Answer from the drawing. Dimensions are ordinates in mm from the lowest x, y and z of the part. Give positions to 0.01 mm unless a question says otherwise; leave off trailing zeros. Order: outer loops, then holes, each group sorted by start corner. A loop starts at its lowest first (then second) coordinate and runs counter-clockwise, first axis right, second up.
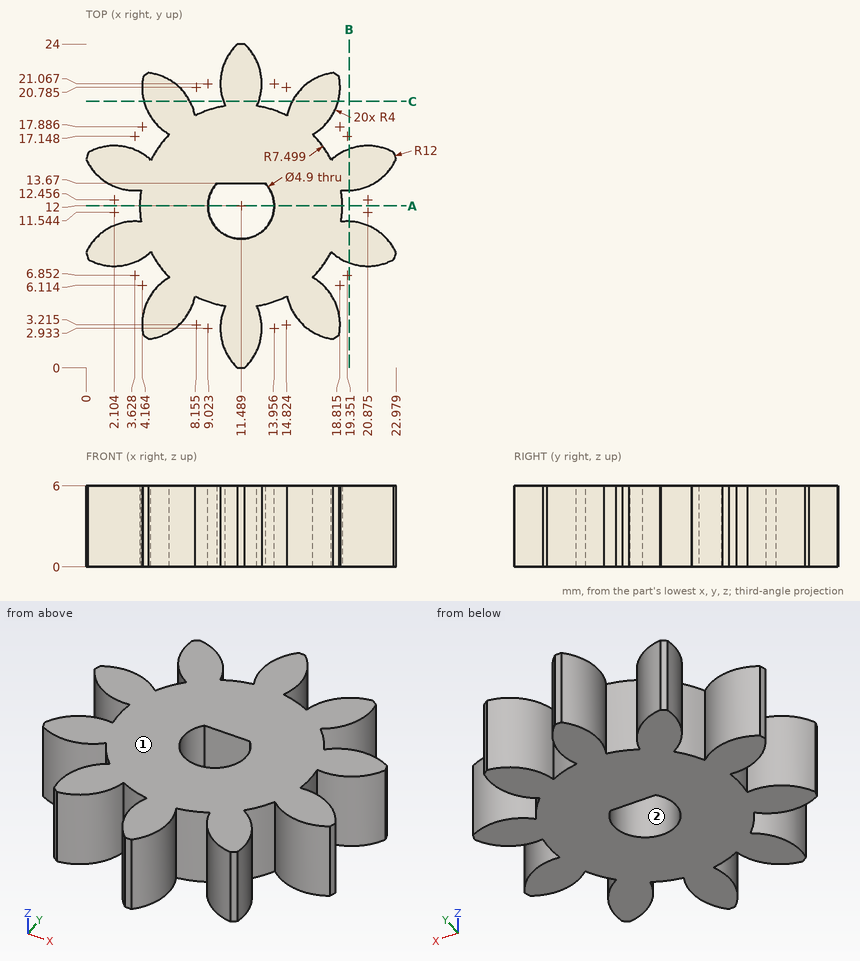
1) Given pin 1 (3 mm diameter, centred on x = 4.5, z = 5, fed in from +Y); pin 2 (1 mm diameter, centred on y = 18, z = 1.5, fed in from -X), each flat-ended and moving along its own axis, determine where each tip first touches the part or whether it passes through.
Final values:
pin 1: stops at y = 21.86
pin 2: stops at x = 4.87
2) For a pull along X with two mould halves and no side action, classify the marked faces 1 and 2 as released by +X, released by -X, zero draft, split by the parting line, or undercut.
Final values:
face 1: zero draft
face 2: undercut
3) Consider L1, parallel to X at y = 5.25, z = 4.05 (1 decimal); L2, parallel to X at y = 3.75, z = 0.65; L3, parallel to Y at x = 9.75, z = 4.85 (1 decimal). Determine where each line is inside the solid, lowest interval first.
Final values:
L1: x = 4.7 to 8.1, 8.2 to 14.8, 14.9 to 18.3
L2: x = 4.19 to 7.39, 10.04 to 12.94, 15.59 to 18.79
L3: y = 4.7 to 10.3, 13.7 to 19.3
4) The part is cut by section B-B on x = 19.5. Determine the outline of the cut face in (y, z).
Final values:
outline: (7.79, 0) - (10.85, 0) - (10.85, 6) - (7.79, 6) - close; (13.15, 0) - (16.21, 0) - (16.21, 6) - (13.15, 6) - close
5) The part is cut by section A-A on y = 12. Determine the outline of the cut face in (x, z).
Final values:
outline: (3.99, 0) - (9.04, 0) - (9.04, 6) - (3.99, 6) - close; (13.94, 0) - (18.99, 0) - (18.99, 6) - (13.94, 6) - close
6) The part is cut by section C-C on y = 19.75. Determine the outline of the cut face in (x, z) (1 decimal).
Final values:
outline: (4.3, 0) - (7.7, 0) - (7.7, 6) - (4.3, 6) - close; (10.2, 0) - (12.8, 0) - (12.8, 6) - (10.2, 6) - close; (15.3, 0) - (18.7, 0) - (18.7, 6) - (15.3, 6) - close
